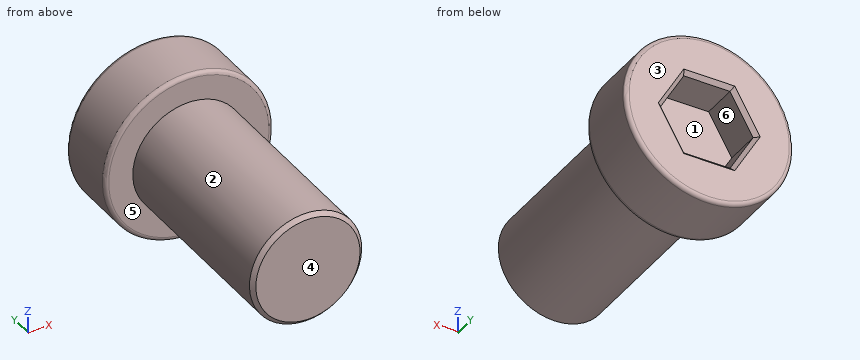
from build123d import *

# Parameters (mm, degrees)
SKETCH_1_R          = 10.5
EXTRUDE_1_DEPTH     = 8
SKETCH_2_R          = 7
EXTRUDE_2_DEPTH     = 25
CUT_EXTRUDE_1_DEPTH = 5
CHAMFER_1_SIZE      = 0.5
FILLET_1_R          = 0.5
CHAMFER_2_SIZE      = 0.5


with BuildPart() as part:
    # 草图1 → 凸台-拉伸1 (new body)
    with BuildSketch(Plane(origin=(0, 0, 0), x_dir=(1, 0, 0), z_dir=(0, 1, 0))):
        with Locations(Location((0, 0, 0), (0, 0, 270))):
            Circle(SKETCH_1_R)
    extrude(amount=EXTRUDE_1_DEPTH)

    # 草图2 → 凸台-拉伸2 (add)
    with BuildSketch(Plane.XZ):
        with Locations(Location((0, 0, 0), (0, 0, 270))):
            Circle(SKETCH_2_R)
    extrude(amount=EXTRUDE_2_DEPTH)

    # 草图3 → 切除-拉伸1 (cut)
    with BuildSketch(Plane(origin=(0, 8, 0), x_dir=(1, 0, 0), z_dir=(0, 1, 0))):
        Polygon((5.773502692, 0), (2.886751346, 5), (-2.886751346, 5), (-5.773502692, 0), (-2.886751346, -5), (2.886751346, -5), align=None)
    extrude(amount=-CUT_EXTRUDE_1_DEPTH, mode=Mode.SUBTRACT)

    # 倒角1
    chamfer_1_edges = [part.edges().sort_by_distance(p)[0] for p in [
        (0, -25, 7),
    ]]
    chamfer(chamfer_1_edges, length=CHAMFER_1_SIZE)

    # 圆角1
    fillet_1_edges = [part.edges().sort_by_distance(p)[0] for p in [
        (0, 0, -10.5),
        (0, 8, -10.5),
    ]]
    fillet(fillet_1_edges, radius=FILLET_1_R)

    # 倒角2
    chamfer_2_edges = [part.edges().sort_by_distance(p)[0] for p in [
        (4.330127019, 8, 2.5),
        (4.330127019, 8, -2.5),
        (0, 8, -5),
        (-4.330127019, 8, -2.5),
        (-4.330127019, 8, 2.5),
        (0, 8, 5),
    ]]
    chamfer(chamfer_2_edges, length=CHAMFER_2_SIZE)


solid = part.part
Work out the finished part from the listing and answer in its coordinate system (mm). Face numbers are marked on the shaded views. A direction names the side the tool comes from. Give positions to 0.01 mm unless a question says otherwise; leave off trailing zeros. Loops run counter-clockwise (first coordinate to the right, second up) from the corner with the lowest first, then second, coordinate; pieces in that order, holes last. Notation, with made-up numbers: (85, 25) -> (120, 25) arc R20 ccw to (120, 34) -> close; hole circle Ø6 at (4.5, 53.5). An arc over 180 degrees is marked (long way). Use a Markdown table: item, result. Add a question column.
1) The part is cut by section B-B, the plane x = 0. Determine the outline of the cut face in (y, z).
2) Each of these flat-tipped pins is pushed along its axis until it touches: P1, Ø10, axis at y = -10.5, z = -6.5, coming from the +X side; P2, Ø1, axis at x = -1.5, z = -1.5, coming from the +Y side; P3, Ø8, axis at y = 0.5, z = 3, coming from the -X side; P4, Ø6, axis at x = -4.5, y = -4.5, coming from the +Z side. Where does it stop, or does it pass through?
3) Consider line 1 along Y through (x, z) = (7, 3.5); line 2 along Y through (x, z) = (2.75, 4.75); line 3 along X through (y, z) = (-16.5, 1.5). Determine where each line is inside the solid, lowest interval first.
4) The part is cut by section A-A, the plane y = 4.5. Determine the outline of the cut face in (x, z), plus the area to 3 significant figures.
5) The part is cut by section C-C, the plane y = -7. Determine the outline of the cut face in (x, z).
6) Which of the six approach directions +Z, -Z, +X, -X, +Y, -Y give full straight-line access (tool end or side, diameter ignored) to the marked faces 4, 5 and 6?
7) For a pull along Z with two mould halves and no side action, classify the marked faces 1, 2 and 3 as +Z half, -Z half, draft (parallel to the pull), parting line (faces both ways), or undercut.
Reported:
| question | item | result |
|---|---|---|
| 1 | outline | (-25, -6.5) -> (-24.5, -7) -> (0, -7) -> (0, -10) arc R0.5 ccw to (0.5, -10.5) -> (7.5, -10.5) arc R0.5 ccw to (8, -10) -> (8, -5.5) -> (7.5, -5) -> (3, -5) -> (3, 5) -> (7.5, 5) -> (8, 5.5) -> (8, 10) arc R0.5 ccw to (7.5, 10.5) -> (0.5, 10.5) arc R0.5 ccw to (0, 10) -> (0, 7) -> (-24.5, 7) -> (-25, 6.5) -> close |
| 2 | P1 | stops at x = 6.84 |
| 2 | P2 | stops at y = 3 |
| 2 | P3 | stops at x = -10.5 |
| 2 | P4 | stops at z = 6.84 |
| 3 | line 1 | y = 0 to 8 |
| 3 | line 2 | y = -25 to 3 |
| 3 | line 3 | x = -6.84 to 6.84 |
| 4 | outline | circle Ø21 at (0, 0); hole (-5.77, 0) -> (-2.89, -5) -> (2.89, -5) -> (5.77, 0) -> (2.89, 5) -> (-2.89, 5) -> close |
| 4 | area | 260 mm^2 |
| 5 | outline | circle Ø14 at (0, 0) |
| 6 | face 4 | +Z, -Z, +X, -X, -Y |
| 6 | face 5 | -Y |
| 6 | face 6 | +Y |
| 7 | face 1 | undercut |
| 7 | face 2 | parting line |
| 7 | face 3 | draft |
